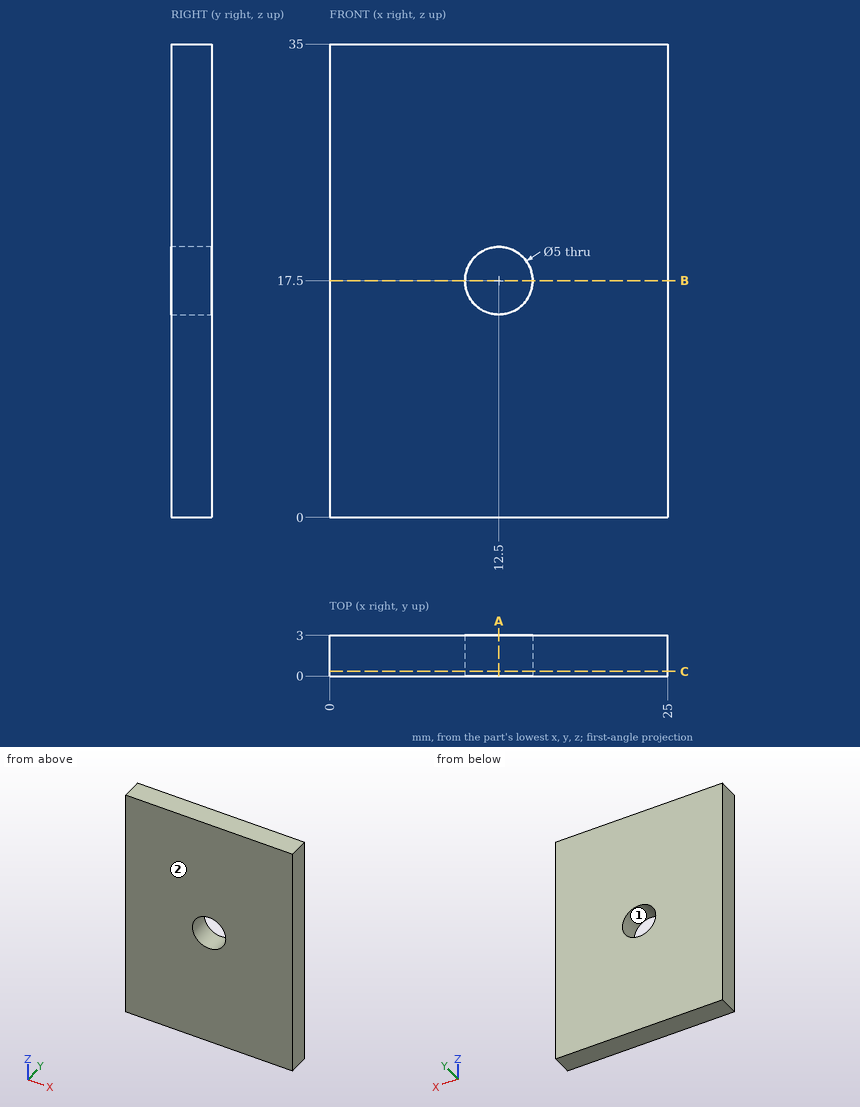
Could you check a few things on this drawing? It's one solid part, dimensions in mm from its lowest x, y, z. Give positions to 0.01 mm unless a question says otherwise; leave off trailing zeros. Order: outer loops, then holes, each group sorted by start corner. A loop starts at its lowest first (then second) coordinate and runs counter-clockwise, first axis right, second up. Notation, with made-up numbers: (-40, 46) - (18, 46) arc R20 ccw to (18, 84) - close; hole circle Ø10 at (77, 38). An arc over 180 degrees is marked (long way). One line per question, with ' | ' between items. Start each with the question number.
Item 1: I need wall thicknesses on probe 1 along Z at (x, y) = (12.5, 1.6); probe 2 along X at (y, z) = (2.05, 17.5); probe 3 along X at (y, z) = (0.5, 15.5). Which ranges of each line are inside material? Lowest first, please. Write a range as [from, to].
Item 2: Thinking about a two-plate mould opening in X: for the marked faces 1 and 2, which applies, pulls with the +X half, pulls with the -X half, needs draft (parallel to the pull), parting line crosses it, or undercut?
Item 3: I want a section at A-A on x = 12.5. Write out the boundary of the cut face in (y, z), then the cut area to 3 significant figures.
Item 4: I want a section at B-B on z = 17.5. Write out the boundary of the cut face in (x, y), then the cut area to 3 significant figures.
Item 5: I want a section at C-C on y = 0.35. Write out the boundary of the cut face in (x, z), then the cut area to 3 significant figures.
Verdict:
1) probe 1: [0, 15], [20, 35] | probe 2: [0, 10], [15, 25] | probe 3: [0, 11], [14, 25]
2) face 1: undercut | face 2: needs draft
3) outline: (0, 0) - (3, 0) - (3, 15) - (0, 15) - close; (0, 20) - (3, 20) - (3, 35) - (0, 35) - close | area: 90.0 mm^2
4) outline: (0, 0) - (10, 0) - (10, 3) - (0, 3) - close; (15, 0) - (25, 0) - (25, 3) - (15, 3) - close | area: 60.0 mm^2
5) outline: (0, 0) - (25, 0) - (25, 35) - (0, 35) - close; hole circle Ø5 at (12.5, 17.5) | area: 855 mm^2
